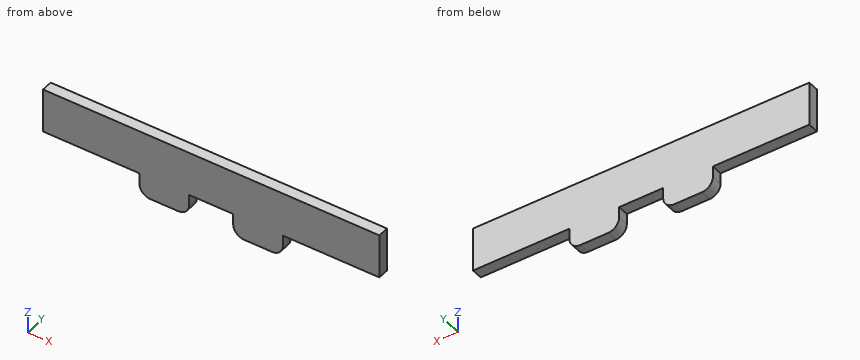
```python
from build123d import *

# Parameters (mm, degrees)
SKETCH1_W           = 45
SKETCH1_H           = 20
SKETCH1_W_2         = 304.8
SKETCH1_H_2         = 40
BOSS_EXTRUDE1_DEPTH = 10
FILLET1_R           = 10


with BuildPart() as part:
    # Sketch1 → Boss-Extrude1 (new body)
    with BuildSketch(Plane(origin=(0, 0, 0), x_dir=(1, 0, 0), z_dir=(0, 1, 0))):
        with Locations((-42.5, 30)):
            Rectangle(SKETCH1_W, SKETCH1_H)
        with Locations((42.5, 30)):
            Rectangle(SKETCH1_W, SKETCH1_H)
        Rectangle(SKETCH1_W_2, SKETCH1_H_2)
    extrude(amount=BOSS_EXTRUDE1_DEPTH)

    # Fillet1
    fillet1_edges = [part.edges().sort_by_distance(p)[0] for p in [
        (-20, 5, -40),
        (20, 5, -40),
        (65, 5, -40),
        (-65, 5, -40),
    ]]
    fillet(fillet1_edges, radius=FILLET1_R)


solid = part.part
```
For this review, take the finished solid that the model builds, in its own axes (mm). Round coordinates to 2 decimals unless told otherwise and drop trailing zeros. Write each loop counter-clockwise with the first axis right and the second up, starting at its lowest first coordinate (ties: lowest second). Pieces come first, ordered by that corner, then holes. Notation, with made-up numbers: (57.5, -14.75) -> (94.5, -14.75) arc R21 ccw to (94.5, 0.25) -> close; hole circle Ø9 at (18.25, 36). An arc over 180 degrees is marked (long way). One line per question, with ' | ' between items. Start each with the question number.
(1) Insertion check: P1, Ø5, axis at y = 3.5, z = -23.5, coming from the -X side; P2, Ø1.5, axis at y = 7.5, z = -23, coming from the +X side. Each pin has a flat end and moves straight along its axis. Give the tip position at first contact, or say it passes through.
(2) Add section A-A, the plane y = 4. Write out the cut boundary in (x, z), plus the area to 3 significant figures.
(3) For line 1 along X through (y, z) = (7.5, -23); line 2 along X through (y, z) = (4.75, -31); line 3 along Z through (x, y) = (67.5, 7.5), list the stretches that pass through material, from the lowest coordinate up. Write a range as from..to.
(4) Add section B-B, the plane x = 5. Write out the cut boundary in (y, z).
Answer list:
1) P1: x = -65 | P2: x = 65
2) outline: (-152.4, -20) -> (-65, -20) -> (-65, -30) arc R10 ccw to (-55, -40) -> (-30, -40) arc R10 ccw to (-20, -30) -> (-20, -20) -> (20, -20) -> (20, -30) arc R10 ccw to (30, -40) -> (55, -40) arc R10 ccw to (65, -30) -> (65, -20) -> (152.4, -20) -> (152.4, 20) -> (-152.4, 20) -> close | area: 13,900 mm²
3) line 1: -65..-20, 20..65 | line 2: -64.95..-20.05, 20.05..64.95 | line 3: -20..20
4) outline: (0, -20) -> (10, -20) -> (10, 20) -> (0, 20) -> close
